The drawing under review shows one solid part. Ordinate dimensions are in mm from its lowest x, y, z. Round coordinates to 2 decimals unless told otherwise and drop trailing zeros. Order: outer loops, then holes, each group sorted by start corner. A loop starts at its lowest first (then second) coordinate and runs counter-clockwise, first axis right, second up.
1) Consider section B-B (x = 0.65). Give the number of separate pieces and of enclosed holes in the cut face, then the cut area to 3 significant figures.
2) Clearance check with flat-ended pins moving along their axes: P1, Ø1, axis at x = 2.5, y = 55, coming from the -Z side (1 decimal); P2, Ø1, axis at x = 1, y = 39, coming from the +Z side. State where each tip first meets the part, or that it passes through.
3) To check wall thickness, follow L1, parallel to Y at x = 0.2, z = 58 (1 decimal); L2, parallel to Y at x = 3, z = 57 (1 decimal); L3, parallel to Y at x = 2.8, z = 23. State the ranges of each line that lie inside material, in increasing order.
4) Consider section D-D (y = 25). Give the boundary of the cut face in (x, z) (1 decimal), then the cut area to 3 significant figures.
5) Consider section A-A (z = 52). Give the boundary of the cut face in (x, y) (1 decimal), then the cut area to 3 significant figures.
6) Consider section C-C (z = 24.5). Give the boundary of the cut face in (x, y) (1 decimal).
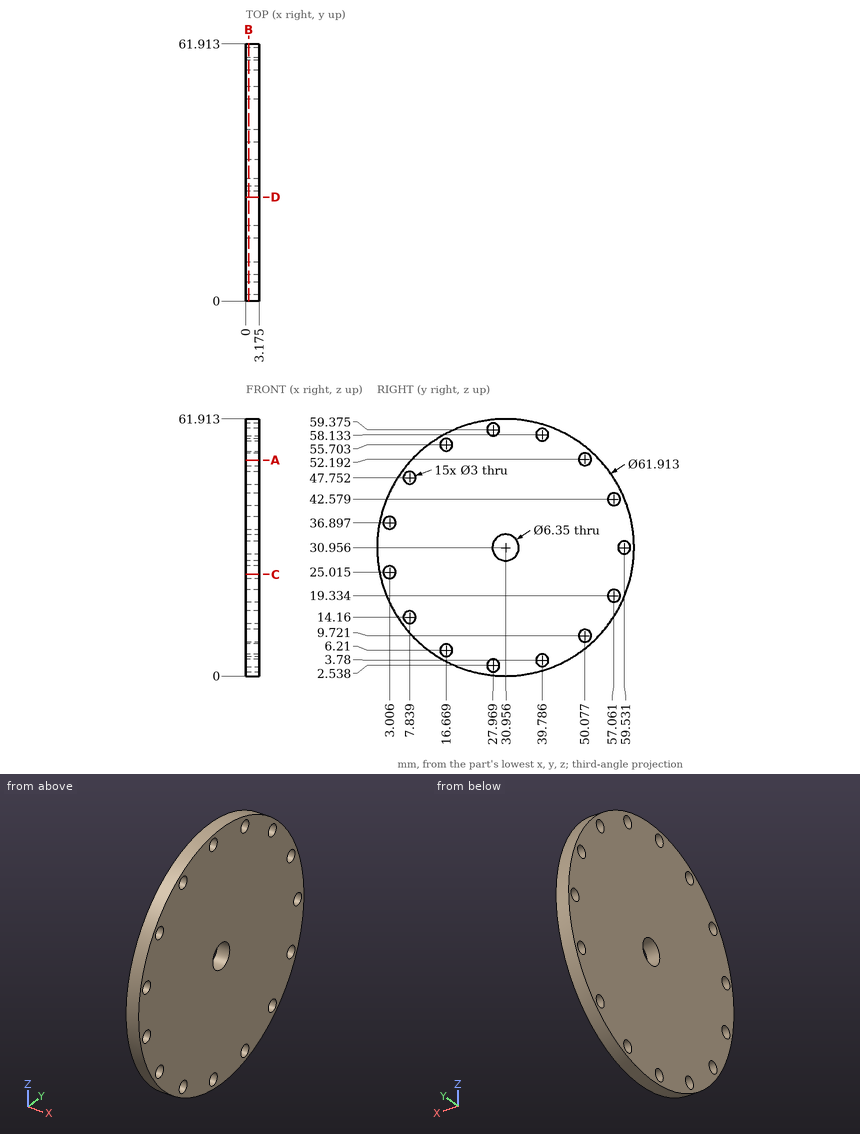
Answer below:
1. separate pieces: 1
1. enclosed holes: 16
1. area: 2,870 mm2
2. P1: stops at z = 10.9
2. P2: stops at z = 60.98
3. L1: y = 15.9 to 27.4, 28.6 to 38.3, 41.3 to 46
3. L2: y = 14.2 to 15.9, 17.4 to 38.8, 40.8 to 47.7
3. L3: y = 1.04 to 60.87
4. outline: (0, 0.6) - (3.2, 0.6) - (3.2, 61.3) - (0, 61.3) - close
4. area: 193 mm2
5. outline: (0, 8.3) - (3.2, 8.3) - (3.2, 48.6) - (0, 48.6) - close; (0, 51.6) - (3.2, 51.6) - (3.2, 53.7) - (0, 53.7) - close
5. area: 135 mm2
6. outline: (0, 0.7) - (3.2, 0.7) - (3.2, 1.6) - (0, 1.6) - close; (0, 4.4) - (3.2, 4.4) - (3.2, 61.2) - (0, 61.2) - close
